Read the model definition and answer for the solid it produces. Units are mm, in the model's axes. A direction names the side the tool comes from. Give positions to 0.01 mm unless a question says otherwise; leave off trailing zeros. Loops run counter-clockwise (first coordinate to the right, second up) from the corner with the lowest first, then second, coordinate; pieces in that order, holes last. Notation, with made-up numbers: M -25,47 L -19,47 A21 cw -19,51 Z; hole C 21,17 d11. An arc over 180 degrees is marked long. Return JSON: item names as keys, results as strings. Group by question number.
```python
from build123d import *

# Parameters (mm, degrees)
SKETCH1_W                = 140
SKETCH1_H                = 150
BODY_DEPTH               = 4
MOUNTING_HOLES_OUTLINE_R = 2.25
MOUNTING_HOLES_DEPTH     = 4
SKETCH5_W                = 140
SKETCH5_H                = 20
CABLE_CANAL_DEPTH        = 1


# Read off the part's stored shape, not the designer's step: mounting_holes
with BuildPart() as part:
    # Sketch1 → body (new body)
    with BuildSketch(Plane(origin=(0, 0, 0), x_dir=(1, 0, 0), z_dir=(0, 1, 0))):
        Rectangle(SKETCH1_W, SKETCH1_H)
    extrude(amount=BODY_DEPTH)

    # mounting_holes outline → mounting_holes (cut)
    with BuildSketch(Plane(origin=(0, 0, 0), x_dir=(1, 0, 0), z_dir=(0, 1, 0))):
        with Locations((65, 70)):
            Circle(MOUNTING_HOLES_OUTLINE_R)
        with Locations((-65, -70)):
            Circle(MOUNTING_HOLES_OUTLINE_R)
        with Locations((65, -70)):
            Circle(MOUNTING_HOLES_OUTLINE_R)
        with Locations((-65, 70)):
            Circle(MOUNTING_HOLES_OUTLINE_R)
    extrude(amount=MOUNTING_HOLES_DEPTH, mode=Mode.SUBTRACT)

    # Sketch5 → cable_canal (cut)
    with BuildSketch(Plane(origin=(0, 4, 0), x_dir=(1, 0, 0), z_dir=(0, 1, 0))):
        with Locations((0, 15)):
            Rectangle(SKETCH5_W, SKETCH5_H)
    extrude(amount=-CABLE_CANAL_DEPTH, mode=Mode.SUBTRACT)


solid = part.part
```
1. Find section C-C (x = -43.5). Write down the section's boundary in (y, z), and give its area (3 significant figures).
2. For faces 1 (the cylindrical face through (-65.488, 1.972, 72.196)), 2 (the flat face through (-1, 3, -15)), determine the directions among +Z, -Z, +X, -X, +Y, -Y from which every point of the face is accessible in a straight line to the end or side of a thin tool.
3. Find section A-A (x = -65). Write down the section's boundary in (y, z).
4. Find section B-B (z = 70). Write down the section's boundary in (x, y).
5. Flat-ended cylindrical pins translate along their axes: P1, Ø3.5, axis at x = -65, z = 70, coming from the -Y side; P2, Ø6, axis at x = 10.5, z = -17.5, coming from the +Y side. Find the tip coordinate at first contact, or state that the pin passes through.
6. Straight lines are drawn through the part: line 1 along X through (y, z) = (1.3, 70); line 2 along Z through (x, y) = (65, 1.05); line 3 along Z through (x, y) = (-20, 3.25). For each, find the intervals that lie inside material, in ascending order.
7. The mould has two halves that part along Z. Classify faces 3 (the cylindrical face through (-65.488, 1.972, -67.804)), 4 (the flat face through (-1, 4, 34)), 5 (the flat face through (-1, 2, 75)): +Z half, -Z half, draft (parallel to the pull), parting line (faces both ways), or undercut.
Result:
{
 "1": {"outline": "M 0,-75 L 4,-75 L 4,-25 L 3,-25 L 3,-5 L 4,-5 L 4,75 L 0,75 Z", "area": "580 mm2"},
 "2": {"face 1": "+Y, -Y", "face 2": "+X, -X, +Y"},
 "3": {"outline": "M 0,-75 L 4,-75 L 4,-72.25 L 0,-72.25 Z; M 0,-67.75 L 4,-67.75 L 4,-25 L 3,-25 L 3,-5 L 4,-5 L 4,67.75 L 0,67.75 Z; M 0,72.25 L 4,72.25 L 4,75 L 0,75 Z"},
 "4": {"outline": "M -70,0 L -67.25,0 L -67.25,4 L -70,4 Z; M -62.75,0 L 62.75,0 L 62.75,4 L -62.75,4 Z; M 67.25,0 L 70,0 L 70,4 L 67.25,4 Z"},
 "5": {"P1": "passes through", "P2": "stops at y = 3"},
 "6": {"line 1": "x = -70 to -67.25, -62.75 to 62.75, 67.25 to 70", "line 2": "z = -75 to -72.25, -67.75 to 67.75, 72.25 to 75", "line 3": "z = -75 to -25, -5 to 75"},
 "7": {"face 3": "undercut", "face 4": "draft", "face 5": "+Z half"}
}
